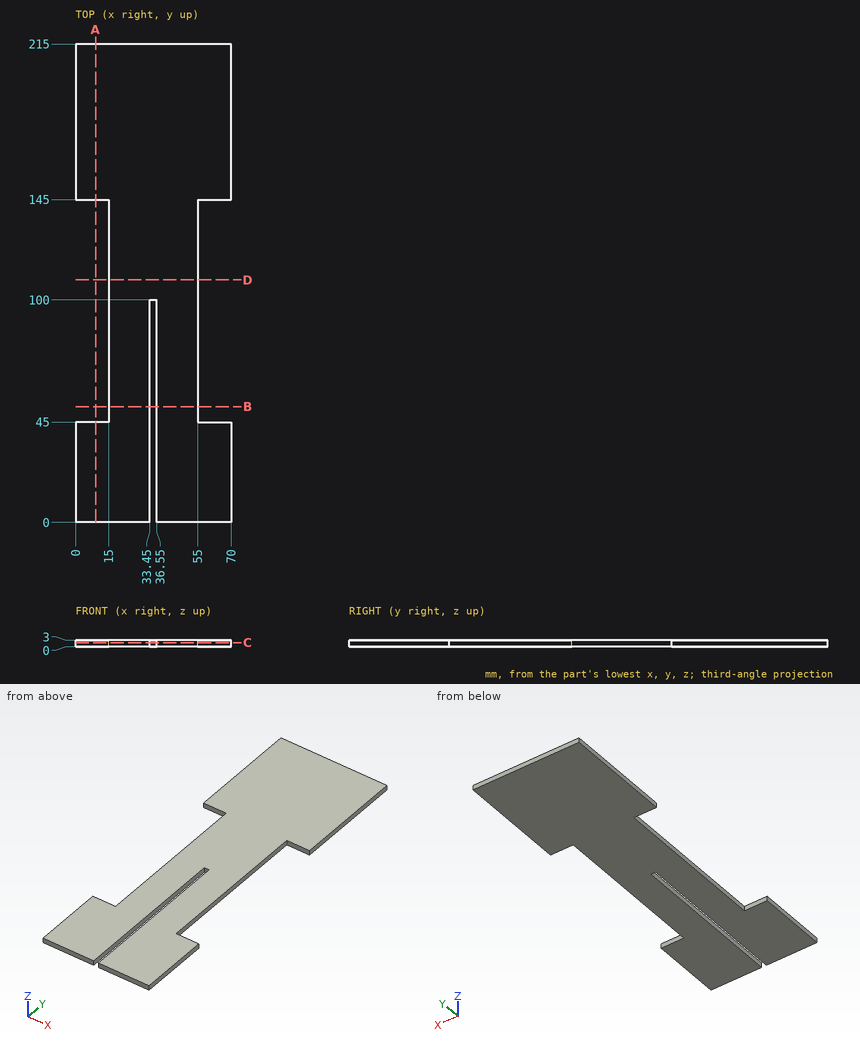
Job drawing, mm, ordinate dimensions from the low corner. One solid piece. Give positions to 0.01 mm unless a question says otherwise; leave off trailing zeros. Write each loop counter-clockwise with the first axis right and the second up, starting at its lowest first coordinate (ties: lowest second). Pieces come first, ordered by that corner, then holes. Notation, with made-up numbers: (24, -7.5) - (52, -7.5) arc R16 ccw to (52, 14.5) - close; hole circle Ø10 at (-24, 12). An arc over 180 degrees is marked (long way). Answer as CSV lines item,"result".
1. Band-saw the part on A-A (x = 9). Write the cut outline in (y, z).
Responses:
outline,"(0, 0) - (45, 0) - (45, 3) - (0, 3) - close; (145, 0) - (215, 0) - (215, 3) - (145, 3) - close"
2. Band-saw the part on B-B (y = 52). Write the cut outline in (x, z).
Responses:
outline,"(15, 0) - (33.45, 0) - (33.45, 3) - (15, 3) - close; (36.55, 0) - (55, 0) - (55, 3) - (36.55, 3) - close"
3. Pin check, flat tips, straight feed: pin 1 (0.9 mm diameter, centred on y = 93.5, z = 2, fed in from -X); pin 2 (0.9 mm diameter, centred on y = 109.5, z = 1.5, fed in from +X). Stop position of each tip, or through.
Responses:
pin 1,"stops at x = 15"
pin 2,"stops at x = 55"
4. Band-saw the part on C-C (z = 2). Write the cut outline in (x, y), and give its area (3 significant figures).
Responses:
outline,"(0, 0) - (33.45, 0) - (33.45, 100) - (36.55, 100) - (36.55, 0) - (70, 0) - (70, 45) - (55, 45) - (55, 145) - (70, 145) - (70, 215) - (0, 215) - (0, 145) - (15, 145) - (15, 45) - (0, 45) - close"
area,"11,700 mm2"
5. Drill centre lines: L1, parallel to Y at x = 12.5, z = 0.7; L2, parallel to X at y = 94.5, z = 2.45; L3, parallel to X at y = 30, z = 1.8. Where is each one in solid material? Low to high. Write a range as [from, to].
Responses:
L1,"y = [0, 45], [145, 215]"
L2,"x = [15, 33.45], [36.55, 55]"
L3,"x = [0, 33.45], [36.55, 70]"
6. Band-saw the part on D-D (y = 109). Write the cut outline in (x, z).
Responses:
outline,"(15, 0) - (55, 0) - (55, 3) - (15, 3) - close"
